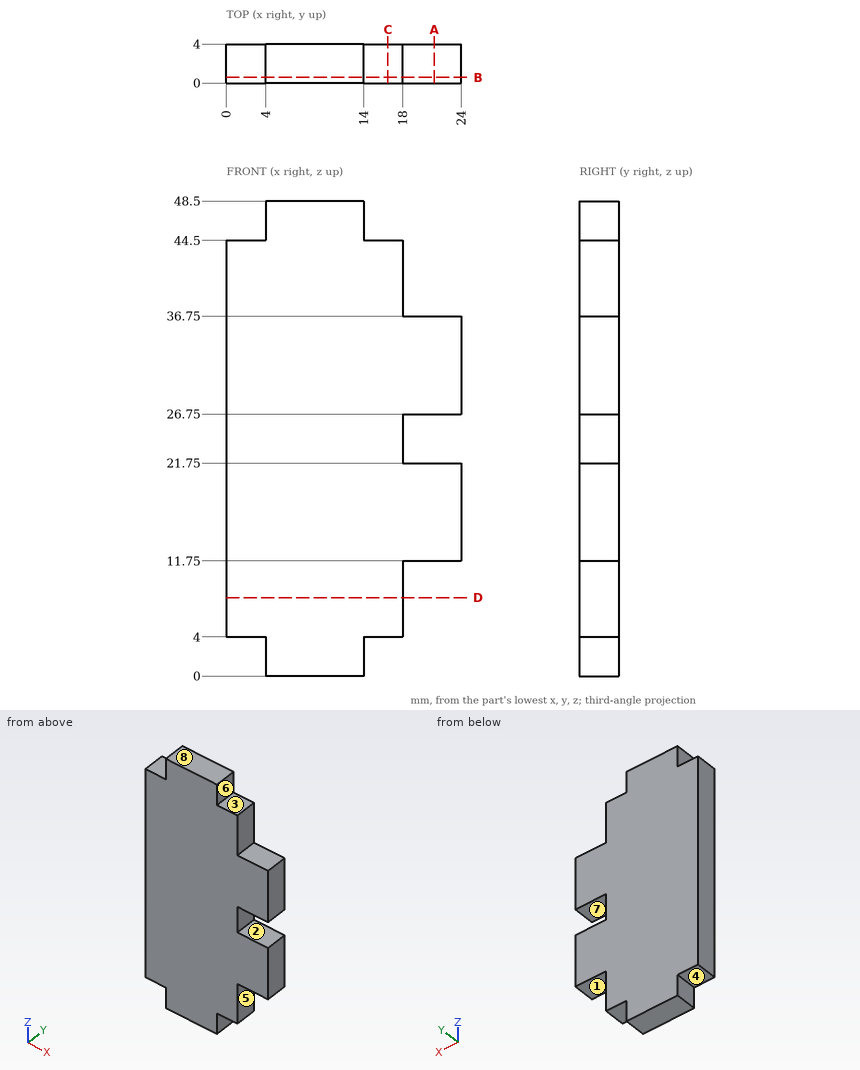
Input: dimensioned drawing with shaded views. Units: mm. Origin: part minimum x, y, z. A direction names the side the tool comes from. Coordinates: 2 decimals unless noted, no trailing zeros. Order: outer loops, then holes, each group sorted by start corner. A loop starts at its lowest first (then second) coordinate and runs counter-clockwise, first axis right, second up. Notation, with made-up numbers: (-21.5, 23) -> (6.5, 23) arc R14 ccw to (6.5, 46) -> close; hole circle Ø3 at (33, 21). An arc over 180 degrees is marked (long way). Answer in a Markdown table with one row per item.
Item 1: Section C-C on x = 16.5. Output: boundary loops of the cut face in (y, z).
Return value:
| item | result |
|---|---|
| outline | (0, 4) -> (4, 4) -> (4, 44.5) -> (0, 44.5) -> close |
Item 2: Access query for the marked faces 4, 5, 6, 7 and 8. Directions: +Z, -Z, +X, -X, +Y, -Y. A direction counts if a zero-diameter tool reaches every point of the face in a straight line with its end or side. Return the directions, or none.
Return value:
| item | result |
|---|---|
| face 4 | -Z, -X, +Y, -Y |
| face 5 | -Z, +X, +Y, -Y |
| face 6 | +Z, +X, +Y, -Y |
| face 7 | +X, +Y, -Y |
| face 8 | +Z, +X, -X, +Y, -Y |
Item 3: Contact query for flat-ended pins moving along their axis: P1, Ø1.2, axis at y = 2, z = 2.5, coming from the +X side; P2, Ø2, axis at y = 2.5, z = 7, coming from the +X side; P3, Ø2, axis at y = 1.5, z = 1.5, coming from the -X side; P4, Ø1.5, axis at y = 1.5, z = 41.5, coming from the -X side. Output: stop coordinate, or through.
Return value:
| item | result |
|---|---|
| P1 | stops at x = 14 |
| P2 | stops at x = 18 |
| P3 | stops at x = 4 |
| P4 | stops at x = 0 |
Item 4: Ray query, L1, parallel to Z at x = 21.75, y = 2.45; L2, parallel to Z at x = 15, y = 0.95; L3, parallel to X at y = 3.75, z = 2. Return the intervals inside material, ascending.
Return value:
| item | result |
|---|---|
| L1 | z = 11.75 to 21.75, 26.75 to 36.75 |
| L2 | z = 4 to 44.5 |
| L3 | x = 4 to 14 |
Item 5: Section A-A on x = 21.25. Output: boundary loops of the cut face in (y, z), plus the area to 3 significant figures.
Return value:
| item | result |
|---|---|
| outline | (0, 11.75) -> (4, 11.75) -> (4, 21.75) -> (0, 21.75) -> close; (0, 26.75) -> (4, 26.75) -> (4, 36.75) -> (0, 36.75) -> close |
| area | 80.0 mm² |
Item 6: Draft query along Z for the marked faces 1, 2 and 3. Return one class per face: released by +Z, released by -Z, zero draft, split by the parting line, or undercut.
Return value:
| item | result |
|---|---|
| face 1 | released by -Z |
| face 2 | undercut |
| face 3 | released by +Z |
Item 7: Section D-D on z = 8. Output: boundary loops of the cut face in (x, y), plus the area to 3 significant figures.
Return value:
| item | result |
|---|---|
| outline | (0, 0) -> (18, 0) -> (18, 4) -> (0, 4) -> close |
| area | 72.0 mm² |
Item 8: Section B-B on y = 0.6. Output: boundary loops of the cut face in (x, z).
Return value:
| item | result |
|---|---|
| outline | (0, 4) -> (4, 4) -> (4, 0) -> (14, 0) -> (14, 4) -> (18, 4) -> (18, 11.75) -> (24, 11.75) -> (24, 21.75) -> (18, 21.75) -> (18, 26.75) -> (24, 26.75) -> (24, 36.75) -> (18, 36.75) -> (18, 44.5) -> (14, 44.5) -> (14, 48.5) -> (4, 48.5) -> (4, 44.5) -> (0, 44.5) -> close |
